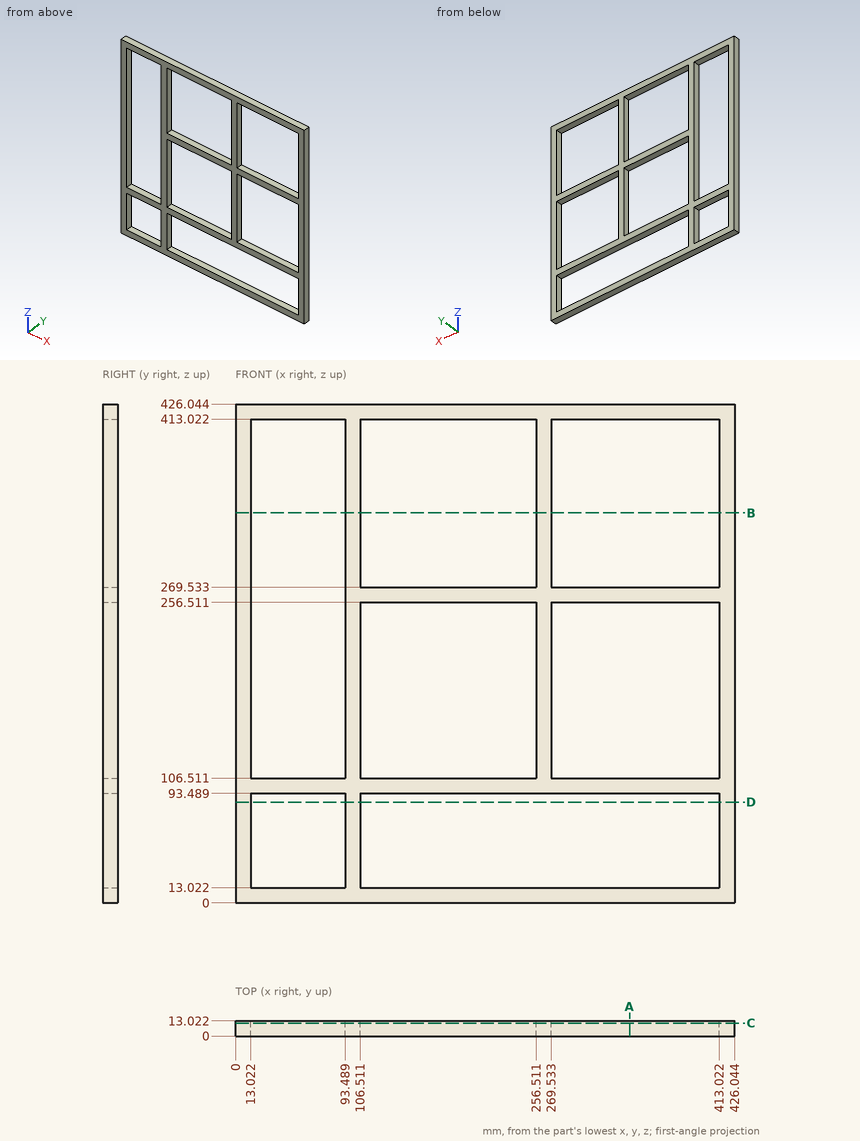
Can you work these out from the drawing? Everything is in mm from the part's minimum corner. Round coordinates to 2 decimals unless told otherwise and drop trailing zeros. Write each loop counter-clockwise with the first axis right and the second up, starting at its lowest first coordinate (ties: lowest second). Pieces come first, ordered by that corner, then holes. Notation, with made-up numbers: M 58.5,55 L 114.5,55 A14 cw 114.5,62 Z; hole C -39,19.25 d4. An arc over 180 degrees is marked long. Use a Markdown table: item, result.
Item 1: I want a section at A-A (x = 336.5). List the corners of the cut face in (y, z) for me, and give its area (3 significant figures).
Found:
| item | result |
|---|---|
| outline | M 0,0 L 13.02,0 L 13.02,13.02 L 0,13.02 Z; M 0,93.49 L 13.02,93.49 L 13.02,106.51 L 0,106.51 Z; M 0,256.51 L 13.02,256.51 L 13.02,269.53 L 0,269.53 Z; M 0,413.02 L 13.02,413.02 L 13.02,426.04 L 0,426.04 Z |
| area | 678 mm2 |
Item 2: I want a section at D-D (z = 86). List the corners of the cut face in (x, y) for me.
Found:
| item | result |
|---|---|
| outline | M 0,0 L 13.02,0 L 13.02,13.02 L 0,13.02 Z; M 93.49,0 L 106.51,0 L 106.51,13.02 L 93.49,13.02 Z; M 413.02,0 L 426.04,0 L 426.04,13.02 L 413.02,13.02 Z |
Item 3: If I drill on line 1 along X through (y, z) = (7.75, 330.5); line 2 along Z through (x, y) = (42, 1.75), over which ranges is the centre line in solid material (lowest first)? Write a range as [from, to].
Found:
| item | result |
|---|---|
| line 1 | x = [0, 13.02], [93.49, 106.51], [256.51, 269.53], [413.02, 426.04] |
| line 2 | z = [0, 13.02], [93.49, 106.51], [413.02, 426.04] |
Item 4: I want a section at C-C (y = 11). State how many separate pieces and enclosed holes the cut face has, and give its area (3 significant figures).
Found:
| item | result |
|---|---|
| separate pieces | 1 |
| enclosed holes | 7 |
| area | 39,600 mm2 |
Item 5: I want a section at B-B (z = 333). List the corners of the cut face in (x, y) for me, and give its area (3 significant figures).
Found:
| item | result |
|---|---|
| outline | M 0,0 L 13.02,0 L 13.02,13.02 L 0,13.02 Z; M 93.49,0 L 106.51,0 L 106.51,13.02 L 93.49,13.02 Z; M 256.51,0 L 269.53,0 L 269.53,13.02 L 256.51,13.02 Z; M 413.02,0 L 426.04,0 L 426.04,13.02 L 413.02,13.02 Z |
| area | 678 mm2 |
